Read the model definition and answer for the solid it produces. Units are mm, in the model's axes. Coordinates: 2 decimals unless noted, no trailing zeros. Order: outer loops, then holes, each group sorted by start corner. A loop starts at its lowest first (then second) coordinate and runs counter-clockwise, first axis right, second up. Notation, with made-up numbers: (41, 69) - (97, 69) arc R19 cw to (97, 98) - close; hole circle Ø10 at (78.25, -37.75). An arc over 180 degrees is marked (long way). Use one line per item in the form item = value.
```python
from build123d import *

# Parameters (mm, degrees)
SKETCH1_R           = 1.6
BOSS_EXTRUDE1_DEPTH = 8
CHAMFER1_SIZE       = 1


with BuildPart() as part:
    # Sketch1 → Boss-Extrude1 (new body)
    with BuildSketch(Plane.XY):
        with BuildLine():
            Line((-0.5, 3), (45.5, 3))
            ThreePointArc((45.5, 3), (47.267766953, 2.267766953), (48, 0.5))
            Line((48, 0.5), (48, -0.5))
            ThreePointArc((48, -0.5), (47.267766953, -2.267766953), (45.5, -3))
            Line((45.5, -3), (-0.5, -3))
            ThreePointArc((-0.5, -3), (-2.267766953, -2.267766953), (-3, -0.5))
            Line((-3, -0.5), (-3, 0.5))
            ThreePointArc((-3, 0.5), (-2.267766953, 2.267766953), (-0.5, 3))
        make_face()
        Circle(SKETCH1_R, mode=Mode.SUBTRACT)
        with Locations((7.5, 0)):
            Circle(SKETCH1_R, mode=Mode.SUBTRACT)
        with Locations((15, 0)):
            Circle(SKETCH1_R, mode=Mode.SUBTRACT)
        with Locations((22.5, 0)):
            Circle(SKETCH1_R, mode=Mode.SUBTRACT)
        with Locations((30, 0)):
            Circle(SKETCH1_R, mode=Mode.SUBTRACT)
        with Locations((37.5, 0)):
            Circle(SKETCH1_R, mode=Mode.SUBTRACT)
        with Locations((45, 0)):
            Circle(SKETCH1_R, mode=Mode.SUBTRACT)
    extrude(amount=BOSS_EXTRUDE1_DEPTH)

    # Chamfer1
    chamfer1_edges = [part.edges().sort_by_distance(p)[0] for p in [
        (-1.6, 0, 0),
        (-1.6, 0, 8),
        (5.9, 0, 0),
        (5.9, 0, 8),
        (13.4, 0, 0),
        (13.4, 0, 8),
        (20.9, 0, 0),
        (20.9, 0, 8),
        (28.4, 0, 0),
        (28.4, 0, 8),
        (35.9, 0, 0),
        (35.9, 0, 8),
        (43.4, 0, 0),
        (43.4, 0, 8),
    ]]
    chamfer(chamfer1_edges, length=CHAMFER1_SIZE)


solid = part.part
```
(1) Given pin 1 Ø3.5 at (x, y) = (37.5, 0) entering from -Z; pin 2 Ø3.5 at (x, y) = (15, 0) entering from +Z; pin 3 Ø2.5 at (x, y) = (30, 0) entering from -Z (3 decimals); pin 4 Ø3 at (y, z) = (-1, 3) entering from -X, each flat-ended and moving along its own axis, determine where each tip first touches the part or whether it passes through.
Answer list:
pin_1 = 0.85
pin_2 = 7.15
pin_3 = through
pin_4 = -3
(2) Section D-D, the plane z = 0.5 is taken. Write down the section's boundary in (x, y), then the cut area to 3 significant figures.
Answer list:
outline = (-3, -0.5) arc R2.5 ccw to (-0.5, -3) - (45.5, -3) arc R2.5 ccw to (48, -0.5) - (48, 0.5) arc R2.5 ccw to (45.5, 3) - (-0.5, 3) arc R2.5 ccw to (-3, 0.5) - close; hole circle Ø4.2 at (0, 0); hole circle Ø4.2 at (7.5, 0); hole circle Ø4.2 at (15, 0); hole circle Ø4.2 at (22.5, 0); hole circle Ø4.2 at (30, 0); hole circle Ø4.2 at (37.5, 0); hole circle Ø4.2 at (45, 0)
area = 204 mm2
(3) Section B-B, the plane x = 37.5 is taken. Write down the section's boundary in (y, z).
Answer list:
outline = (-3, 0) - (-2.6, 0) - (-1.6, 1) - (-1.6, 7) - (-2.6, 8) - (-3, 8) - close; (1.6, 1) - (2.6, 0) - (3, 0) - (3, 8) - (2.6, 8) - (1.6, 7) - close
(4) Section C-C, the plane y = 0 is taken. State how many separate pieces and enclosed holes the cut face has, then the cut area to 3 significant figures.
Answer list:
separate_pieces = 8
enclosed_holes = 0
area = 215 mm2
(5) Straight lines are drawn through the part: L1, parallel to Y at x = 0, z = 3.8; L2, parallel to Y at x = 44, z = 6.25; L3, parallel to X at y = -2.05, z = 0.75. For each, find the intervals that lie inside material, in ascending order.
Answer list:
L1 = -3 to -1.6, 1.6 to 3
L2 = -3 to -1.25, 1.25 to 3
L3 = -2.46 to 47.46
(6) Section A-A, the plane z = 4.25 is taken. Write down the section's boundary in (x, y), then the cut area to 3 significant figures.
Answer list:
outline = (-3, -0.5) arc R2.5 ccw to (-0.5, -3) - (45.5, -3) arc R2.5 ccw to (48, -0.5) - (48, 0.5) arc R2.5 ccw to (45.5, 3) - (-0.5, 3) arc R2.5 ccw to (-3, 0.5) - close; hole circle Ø3.2 at (0, 0); hole circle Ø3.2 at (7.5, 0); hole circle Ø3.2 at (15, 0); hole circle Ø3.2 at (22.5, 0); hole circle Ø3.2 at (30, 0); hole circle Ø3.2 at (37.5, 0); hole circle Ø3.2 at (45, 0)
area = 244 mm2
(7) The mould has two halves that part along X. Classify faces 1 (the cylindrical face through (28.4, 0.07, 3.96)), 2 (the flat face through (28.5, 2.7, 0)), 3 (the flat face through (48, 0, 4)): +X half, -X half, draft (parallel to the pull), parting line (faces both ways), or undercut.
Answer list:
face_1 = undercut
face_2 = draft
face_3 = +X half
